from build123d import *

# Parameters (mm, degrees)
F0_W     = 38.1
F0_H     = 31.75
F1_DEPTH = 25.4
F2_W     = 25.4
F2_H     = 6.35
F3_DEPTH = 25.4
F4_DEPTH = 6.35
F6_DEPTH = 31.75
F7_DEPTH = 57.15
F8_DEPTH = 25.4


with BuildPart() as f1:
    # F0 (on Front) → F1 (new body)
    with BuildSketch(Plane.XZ):
        with Locations((-40.7485894724, 15.875)):
            Rectangle(F0_W, F0_H)
    extrude(amount=F1_DEPTH)

    # F2 (on face) → F3 (cut)
    with BuildSketch(Plane.XY.offset(31.75)):
        with Locations((-34.3985894724, -22.225)):
            Rectangle(F2_W, F2_H)
    extrude(amount=-F3_DEPTH, mode=Mode.SUBTRACT)

    # F4 (cut): a face of the model
    f4_faces = [f1.faces().sort_by_distance(p)[0] for p in [
        (-34.3985894724, -22.225, 6.35),
    ]]
    extrude(f4_faces, amount=-F4_DEPTH, mode=Mode.SUBTRACT)

    # F5 (on face) → F6 (join)
    with BuildSketch(Plane.XY.offset(31.75)):
        Polygon((-47.0985894724, -6.2670672635), (-21.6985894724, -6.2670672635), (-21.6985894724, 0), (-46.0756682071, 0), align=None)
    extrude(amount=F6_DEPTH)

    # F7 (cut): a face of the model
    f7_faces = [f1.faces().sort_by_distance(p)[0] for p in [
        (-34.1446109127, -3.1549983853, 63.5),
    ]]
    extrude(f7_faces, amount=-F7_DEPTH, mode=Mode.SUBTRACT)

    # F8 (cut): a face of the model
    f8_faces = [f1.faces().sort_by_distance(p)[0] for p in [
        (-34.1446109127, -3.1549983853, 6.35),
    ]]
    extrude(f8_faces, amount=-F8_DEPTH, mode=Mode.SUBTRACT)


solid = f1.part
The listing builds one solid part. Answer for the finished solid, in the listing's coordinates (mm). A direction names the side the tool comes from. Give positions to 0.01 mm unless a question says otherwise; leave off trailing zeros. Write each loop counter-clockwise with the first axis right and the second up, starting at its lowest first coordinate (ties: lowest second). Pieces come first, ordered by that corner, then holes.
Item 1: Section C-C, the plane x = -34.5 is taken. Write down the section's boundary in (y, z).
Item 2: Flat-ended cylindrical pins translate along their axes: P1, Ø1.9, axis at y = -23.5, z = 16, coming from the +X side; P2, Ø1.5, axis at x = -44, z = 18, coming from the -Y side; P3, Ø10, axis at x = -34.5, z = 3.5, coming from the +Y side. Find the tip coordinate at first contact, or state that the pin passes through.
Item 3: Which of the six approach directions +Z, -Z, +X, -X, +Y, -Y give full straight-line access (tool end or side, diameter ignored) to faces 5 (the flat face through (-21.699, -13, 16)), 6 (the flat face through (-35, -19.05, 16))?
Item 4: Section B-B, the plane y = -23.25 is taken. Write down the section's boundary in (x, z), plus the area to 3 significant figures.
Item 5: Section A-A, the plane z = 22 is taken. Write down the section's boundary in (x, y), plus the area to 3 significant figures.
Item 6: Determine the mould class of faces 1 (the flat face through (-53, 0, 16)), 2 (the flat face through (-59.799, -13, 16)), 3 (the flat face through (-54, -25.4, 16)), 4 (the flat face through (-46.58, -3.09, 16.1)) for opening direction Y: released by +Y, released by -Y, zero draft, split by the parting line, or undercut.
Item 7: Find the intervals of material crossed by line 1 along X through (y, z) = (-20.5, 13.5); line 2 along Y through (x, z) = (-25.5, 8); line 3 along X through (y, z) = (-1.75, 18), in increasing order.
Completed:
1. outline: (-19.05, 0) - (-6.27, 0) - (-6.27, 31.75) - (-19.05, 31.75) - close
2. P1: stops at x = -47.1
2. P2: stops at y = -19.05
2. P3: stops at y = -6.27
3. face 5: +Z, -Z, +X, +Y, -Y
3. face 6: +Z, -Z, +X, -Y
4. outline: (-59.8, 0) - (-47.1, 0) - (-47.1, 31.75) - (-59.8, 31.75) - close
4. area: 403 mm2
5. outline: (-59.8, -25.4) - (-47.1, -25.4) - (-47.1, -19.05) - (-21.7, -19.05) - (-21.7, -6.27) - (-47.1, -6.27) - (-46.08, 0) - (-59.8, 0) - close
5. area: 650 mm2
6. face 1: released by +Y
6. face 2: zero draft
6. face 3: released by -Y
6. face 4: undercut
7. line 1: x = -59.8 to -47.1
7. line 2: y = -19.05 to -6.27
7. line 3: x = -59.8 to -46.36
